Build history of the part. All positions in model axes, mm. Face numbers are marked on the shaded views. Coordinates: 2 decimals unless noted, no trailing zeros. Loops run counter-clockwise (first coordinate to the right, second up) from the corner with the lowest first, then second, coordinate; pieces in that order, holes last.
(1) Wall check: L1, parallel to X at y = 19.35, z = 12.5; L2, parallel to Y at x = 65, z = -1.05; L3, parallel to Y at x = 47.5, z = 9.5. Give the ranges that are in metal, low to high.
(2) Slice it at C-C (z = 12.5). Give the cut face in (x, y), and give its area (3 significant figures).
(3) Two-plate mould, pull along Z, no slides. Class the marked faces 1, 2 and 3: pulls with the +Z half, pulls with the -Z half, needs draft (parallel to the pull), parting line crosses it, or undercut.
(4) Slice it at A-A (y = 8). Give the cut face in (x, z), and give its area (3 significant figures).
(5) Flat gauge pins, fed straight in: P1, Ø4, axis at x = 21.5, z = 2.5, coming from the -Y side; P2, Ø2.5, axis at y = 12, z = -1, coming from the -X side. Where does each tip first touch, or does it go through?
(6) Slice it at D-D (x = 39.5). Give the cut face in (y, z), and give its area (3 significant figures).
(7) Slice it at B-B (x = 65). Give the cut face in (y, z).
from build123d import *

# Parameters (mm, degrees)
SKETCH1_W           = 75
SKETCH1_H           = 3
BOSS_EXTRUDE1_DEPTH = 20
SKETCH2_W           = 75
SKETCH2_H           = 17
BOSS_EXTRUDE2_DEPTH = 3
FILLET1_R           = 6
FILLET2_R           = 2
SKETCH3_R           = 2.5
CUT_EXTRUDE1_DEPTH  = 21
SKETCH4_R           = 2.5
CUT_EXTRUDE2_DEPTH  = 4


with BuildPart() as part:
    # Sketch1 → Boss-Extrude1 (new body)
    with BuildSketch(Plane(origin=(0, 0, 0), x_dir=(1, 0, 0), z_dir=(0, 1, 0))):
        with Locations((37.5, 1.5)):
            Rectangle(SKETCH1_W, SKETCH1_H)
    extrude(amount=BOSS_EXTRUDE1_DEPTH)

    # Sketch2 → Boss-Extrude2 (add)
    with BuildSketch(Plane(origin=(0, 20, 0), x_dir=(1, 0, 0), z_dir=(0, 1, 0))):
        Polygon((0, 0), (0, 3), (-5, -17), (0, -17), align=None)
        with Locations((37.5, -8.5)):
            Rectangle(SKETCH2_W, SKETCH2_H)
    extrude(amount=-BOSS_EXTRUDE2_DEPTH)

    # Fillet1
    fillet1_edges = [part.edges().sort_by_distance(p)[0] for p in [
        (-5, 18.5, 17),
    ]]
    fillet(fillet1_edges, radius=FILLET1_R)

    # Fillet2
    fillet2_edges = [part.edges().sort_by_distance(p)[0] for p in [
        (37.5, 20, -3),
        (75, 18.5, 17),
        (37.5, 0, -3),
        (75, 0, -1.5),
        (0, 0, -1.5),
    ]]
    fillet(fillet2_edges, radius=FILLET2_R)

    # Sketch3 → Cut-Extrude1 (cut, through all)
    with BuildSketch(Plane(origin=(0, 20, 0), x_dir=(1, 0, 0), z_dir=(0, 1, 0))):
        with Locations((1.794270235, -12.5)):
            Circle(SKETCH3_R)
    extrude(amount=-CUT_EXTRUDE1_DEPTH, mode=Mode.SUBTRACT)

    # Sketch4 → Cut-Extrude2 (cut, through all)
    with BuildSketch(Plane.XY):
        with Locations((65, 8)):
            Circle(SKETCH4_R)
        with Locations((15, 8)):
            Circle(SKETCH4_R)
    extrude(amount=-CUT_EXTRUDE2_DEPTH, mode=Mode.SUBTRACT)


solid = part.part
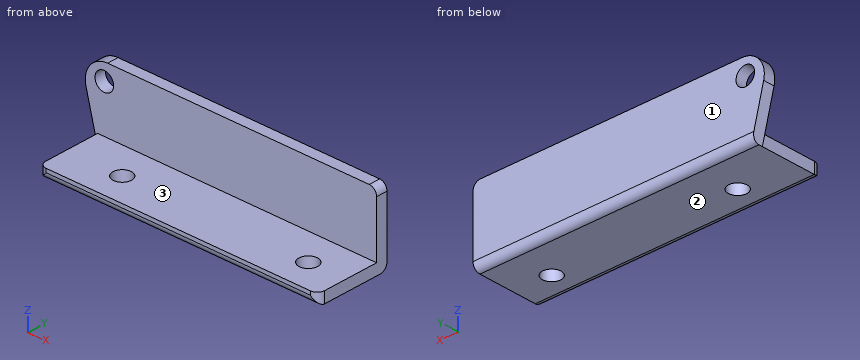
Response values:
1. L1: x = -3.12 to -0.71, 4.29 to 75
1. L2: y = 0 to 5.5, 10.5 to 20
1. L3: y = 17 to 20
2. outline: (-3.12, 17) - (-0.71, 17) - (-0.71, 20) - (-3.12, 20) - close; (4.29, 17) - (75, 17) - (75, 20) - (4.29, 20) - close
2. area: 219 mm2
3. face 1: needs draft
3. face 2: pulls with the -Z half
3. face 3: pulls with the +Z half
4. outline: (0, -3) - (12.5, -3) - (12.5, 0) - (0, 0) - close; (17.5, -3) - (62.5, -3) - (62.5, 0) - (17.5, 0) - close; (67.5, -3) - (75, -3) - (75, 0) - (67.5, 0) - close
4. area: 195 mm2
5. P1: stops at y = 17
5. P2: stops at x = 0
6. outline: (0, -1) arc R2 ccw to (2, -3) - (18, -3) arc R2 ccw to (20, -1) - (20, 17) - (17, 17) - (17, 0) - (0, 0) - close
6. area: 109 mm2
7. outline: (0, -1) arc R2 ccw to (2, -3) - (5.5, -3) - (5.5, 0) - (0, 0) - close; (10.5, -3) - (18, -3) arc R2 ccw to (20, -1) - (20, 17) - (17, 17) - (17, 0) - (10.5, 0) - close
